Study the drawing (mm; zero at the part's minimum x, y, z) and answer. A direction names the side the tool comes from. Give positions to 0.01 mm unless a question says otherwise; leave off trailing zeros. Loops run counter-clockwise (first coordinate to the right, second up) from the corner with the lowest first, then second, coordinate; pieces in that order, holes last. Notation, with made-up numbers: (40, 45.25) - (89, 45.25) arc R7 cw to (89, 53.25) - close; hole circle Ø5 at (48, -4.75). An arc over 180 degrees is marked (long way). Answer in a Markdown table with one row per item. Add a question column.
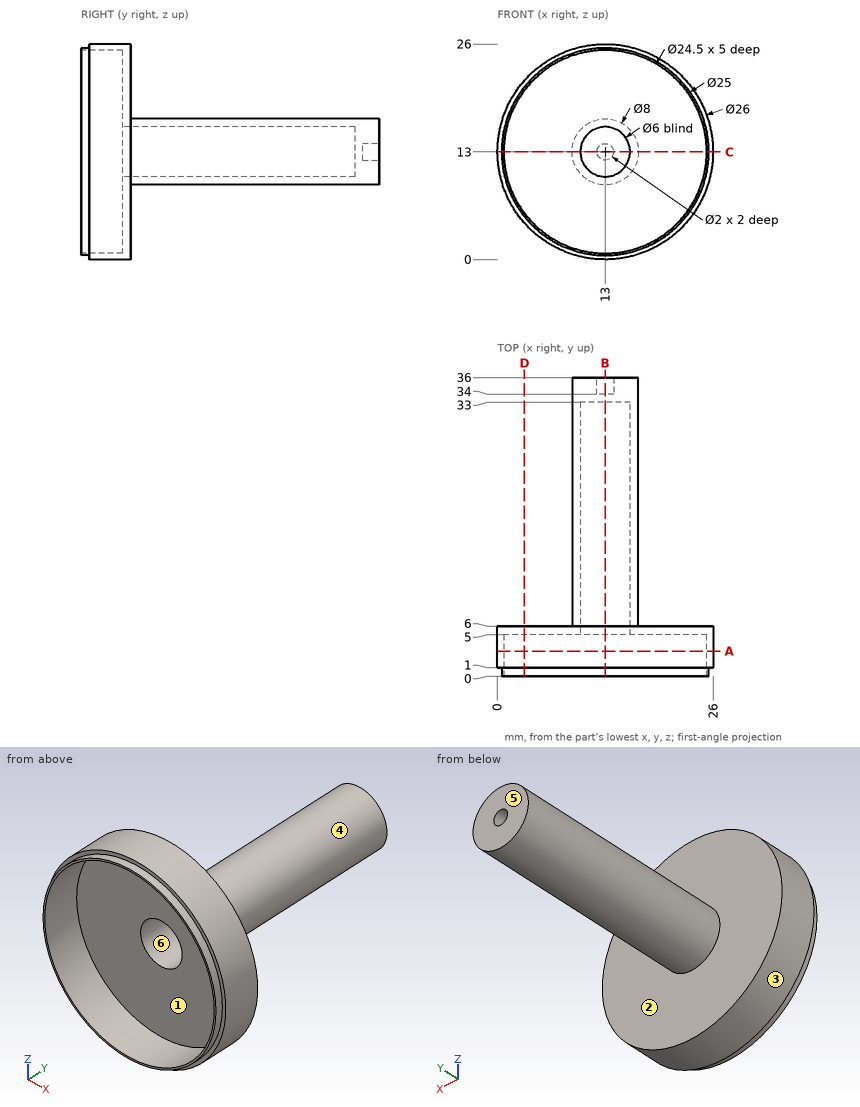
(1) A cutting plane is placed at B-B on x = 13. Determine the outline of the cut face in (y, z), plus the area to 4 significant figures.
(2) A cutting plane is placed at D-D on x = 3.25. Determine the outline of the cut face in (y, z), plus the area to 3 significant figures.
(3) A cutting plane is placed at C-C on z = 13. Determine the outline of the cut face in (x, y).
(4) A cutting plane is placed at A-A on y = 3. Determine the outline of the cut face in (x, z), plus the area to 3 significant figures.
(5) The mould has two halves that part along Z. Classify the marked faces 4, 5 and 6: pulls with the +Z half, pulls with the -Z half, needs draft (parallel to the pull), parting line crosses it, or undercut.
(6) A tool of negligible diameter and unlimited length cuts with its end or side. For the marked faces 1, 2 and 3, from which of +Z, -Z, +X, -X, +Y, -Y can it reach the whole face along a straight path? Write none if from no direction.
(7) Given pin 1 Ø3 at (y, z) = (5, 13.5) entering from -X; pin 2 Ø8 at (x, z) = (8, 16) entering from -Y; pin 3 Ø6 at (x, z) = (6.5, 17.5) entering from +Y; pin 4 Ø1.8 at (x, z) = (13, 13) entering from +Y, each flat-ended and moving along its own axis, determine where each tip first touches the part or whether it passes through.
(8) Find the intervals of material crossed by line 1 along Z through (x, y) = (13, 34.8); line 2 along Z through (x, y) = (13, 19.25); line 3 along Y through (x, z) = (3.25, 17.75), in increasing order. Write a range as [from, to].
Evaluation:
| question | item | result |
|---|---|---|
| 1 | outline | (0, 0.5) - (1, 0.5) - (1, 0) - (6, 0) - (6, 9) - (36, 9) - (36, 12) - (34, 12) - (34, 14) - (36, 14) - (36, 17) - (6, 17) - (6, 26) - (1, 26) - (1, 25.5) - (0, 25.5) - (0, 25.25) - (5, 25.25) - (5, 16) - (33, 16) - (33, 10) - (5, 10) - (5, 0.75) - (0, 0.75) - close |
| 1 | area | 100.5 mm² |
| 2 | outline | (0, 5.18) - (1, 5.18) - (1, 4.4) - (6, 4.4) - (6, 21.6) - (1, 21.6) - (1, 20.82) - (0, 20.82) - (0, 20.42) - (5, 20.42) - (5, 5.58) - (0, 5.58) - close |
| 2 | area | 27.5 mm² |
| 3 | outline | (0, 1) - (0.5, 1) - (0.5, 0) - (0.75, 0) - (0.75, 5) - (10, 5) - (10, 33) - (16, 33) - (16, 5) - (25.25, 5) - (25.25, 0) - (25.5, 0) - (25.5, 1) - (26, 1) - (26, 6) - (17, 6) - (17, 36) - (14, 36) - (14, 34) - (12, 34) - (12, 36) - (9, 36) - (9, 6) - (0, 6) - close |
| 4 | outline | circle Ø26 at (13, 13); hole circle Ø24.5 at (13, 13) |
| 4 | area | 59.5 mm² |
| 5 | face 4 | parting line crosses it |
| 5 | face 5 | needs draft |
| 5 | face 6 | undercut |
| 6 | face 1 | -Y |
| 6 | face 2 | +Y |
| 6 | face 3 | +Y, -Y |
| 7 | pin 1 | stops at x = 0 |
| 7 | pin 2 | stops at y = 5 |
| 7 | pin 3 | stops at y = 6 |
| 7 | pin 4 | stops at y = 34 |
| 8 | line 1 | z = [9, 12], [14, 17] |
| 8 | line 2 | z = [9, 10], [16, 17] |
| 8 | line 3 | y = [5, 6] |
